CAD build for the part. Positions are in the model's coordinates, mm. Face numbers are marked on the shaded views. Coordinates: 2 decimals unless noted, no trailing zeros. Loops run counter-clockwise (first coordinate to the right, second up) from the corner with the lowest first, then second, coordinate; pieces in that order, holes last. Notation, with made-up numbers: (77.25, 84) -> (118.25, 84) arc R10 cw to (118.25, 97) -> close; hole circle Ø4 at (15.25, 70). An arc over 180 degrees is marked (long way). Write each question's results on one line, items separated by ' | '.
```python
from build123d import *


with BuildPart() as part:
    # Çizim1 → Döndür1 (revolve)
    with BuildSketch(Plane.XY, mode=Mode.PRIVATE) as d_nd_r1_sk:
        with BuildLine():
            Line((3.5, 5.4), (3.5, 4.6))
            ThreePointArc((3.5, 4.6), (3.324264069, 4.175735931), (2.9, 4))
            Line((2.9, 4), (-2.9, 4))
            ThreePointArc((-2.9, 4), (-3.324264069, 4.175735931), (-3.5, 4.6))
            Line((-3.5, 4.6), (-3.5, 5.4))
            Line((-3.5, 5.4), (-2, 5.4))
            ThreePointArc((-2, 5.4), (0, 4.636067977), (2, 5.4))
            Line((2, 5.4), (3.5, 5.4))
        make_face()
    revolve(d_nd_r1_sk.sketch.rotate(Axis((-20.148687567, 0, 0), (1, 0, 0)), 90), axis=Axis((-20.148687567, 0, 0), (1, 0, 0)))


solid = part.part
```
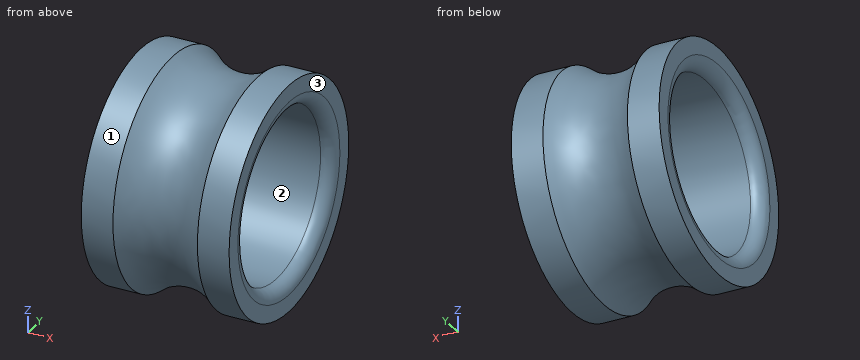
Q1. Cut at D-D on x = 1. Write the cut outline in (y, z), and give its area (3 significant figures).
Results are:
outline: circle Ø9.62 at (0, 0); hole circle Ø8 at (0, 0) | area: 22.3 mm^2
Q2. Wall check: L1, parallel to X at y = 3.75, z = -3.25; L2, parallel to Y at x = -0.45, z = 0; L3, parallel to Y at x = -2.75, z = -1. Give the ranges that are in metal, low to high. Write a range as from..to.
Results are:
L1: -3.5..-1.36, 1.36..3.5 | L2: -4.67..-4, 4..4.67 | L3: -5.31..-3.87, 3.87..5.31
Q3. Pull direction Y, two halves, no side cores. Call the marked faces 1, 2 and 3: +Y half, -Y half, draft (parallel to the pull), parting line (faces both ways), or undercut.
Results are:
face 1: parting line | face 2: undercut | face 3: draft
Q4. Drop flat-ended pins along their axis: pin 1 (1 mm diameter, centred on x = -1.5, y = 3.5, fed in from -Z); pin 2 (1 mm diameter, centred on x = -2.5, y = 1.5, fed in from +Z); pin 3 (1 mm diameter, centred on x = -1, y = 3.5, fed in from -Z); pin 4 (2 mm diameter, centred on y = -1.5, z = 2, fed in from +X). Give the stop position or say it passes through.
Results are:
pin 1: z = -4.24 | pin 2: z = 5.31 | pin 3: z = -3.84 | pin 4: through
Q5. Cut at A-A on z = 0. Write the cut outline in (x, y).
Results are:
outline: (-3.5, -5.4) -> (-2, -5.4) arc R3 cw to (2, -5.4) -> (3.5, -5.4) -> (3.5, -4.6) arc R0.6 ccw to (2.9, -4) -> (-2.9, -4) arc R0.6 ccw to (-3.5, -4.6) -> close; (-3.5, 4.6) arc R0.6 ccw to (-2.9, 4) -> (2.9, 4) arc R0.6 ccw to (3.5, 4.6) -> (3.5, 5.4) -> (2, 5.4) arc R3 cw to (-2, 5.4) -> (-3.5, 5.4) -> close
Q6. Cut at C-C on x = 2.5. Write the cut outline in (y, z).
Results are:
outline: circle Ø10.8 at (0, 0); hole circle Ø8 at (0, 0)
